```python
from build123d import *
from OCP.BRepFilletAPI import BRepFilletAPI_MakeChamfer

# Parameters (mm, degrees)
BOSS_EXTRUDE1_DEPTH       = 25.4
BOSS_EXTRUDE2_DEPTH       = 38.1
F_6_32_TAPPED_HOLE1_D     = 2.7051
F_6_32_TAPPED_HOLE1_DEPTH = 12.7
F_6_32_TAPPED_HOLE1_TIP   = 0.8126940302657266
CHAMFER1_SIZE             = 2.54
BOSS_EXTRUDE3_DEPTH       = 25.4
CHAMFER2_SIZE             = 7.619999999999999
CHAMFER2_SIZE2            = 5.388153672641502


with BuildPart() as part:
    # Sketch1 → Boss-Extrude1 (new body)
    with BuildSketch(Plane.XY):
        Polygon((0, -3.592102448427662), (-16.01038418160373, 12.418281733176066), (-16.010384181603733, 24.90038418160373), (16.01038418160373, 24.90038418160373), (16.010384181603733, 12.418281733176075), align=None)
        Polygon((0, 0), (-13.47038418160373, 13.47038418160373), (-13.470384181603732, 22.360384181603727), (13.470384181603732, 22.360384181603727), (13.47038418160373, 13.47038418160373), align=None, mode=Mode.SUBTRACT)
    extrude(amount=BOSS_EXTRUDE1_DEPTH)

    # Sketch2 → Boss-Extrude2 (add)
    with BuildSketch(Plane.XY.offset(25.4)):
        Polygon((0, 0), (-5.388153672641493, 5.388153672641493), (-7.184204896855324, 3.592102448427661), (0, -3.592102448427662), (7.184204896855322, 3.5921024484276627), (5.388153672641491, 5.3881536726414945), align=None)
    extrude(amount=BOSS_EXTRUDE2_DEPTH)

    # #6-32 Tapped Hole1
    with Locations(Plane(origin=(0, 24.90038418160373, 0), x_dir=(1, 0, 0), z_dir=(0, 1, 0))):
        with Locations((0, -3.175), (0, -22.225)):
            Hole(F_6_32_TAPPED_HOLE1_D / 2, depth=F_6_32_TAPPED_HOLE1_DEPTH)
            with Locations((0, 0, -(F_6_32_TAPPED_HOLE1_DEPTH + F_6_32_TAPPED_HOLE1_TIP / 2))):  # 118° drill point
                Cone(0, F_6_32_TAPPED_HOLE1_D / 2, F_6_32_TAPPED_HOLE1_TIP, mode=Mode.SUBTRACT)

    # Chamfer1
    chamfer1_edges = [part.edges().sort_by_distance(p)[0] for p in [
        (0, -3.592102448427662, 31.75),
    ]]
    chamfer(chamfer1_edges, length=CHAMFER1_SIZE)

    # Sketch5 → Boss-Extrude3 (add)
    with BuildSketch(Plane(origin=(0, 0, 0), x_dir=(-1, 0, 0), z_dir=(0, 0, -1))):
        Polygon((1.7960512242138398, -1.7960512242138225), (-1.7960512242138331, -1.7960512242138298), (-12.29, -1.796051224213831), (-12.289999999999996, -23.336051224213833), (-9.749999999999998, -23.336051224213833), (-9.749999999999998, -4.336051224213831), (9.749999999999998, -4.336051224213828), (9.750000000000005, -23.33605122421383), (12.290000000000003, -23.33605122421383), (12.29, -1.796051224213828), align=None)
    extrude(amount=-BOSS_EXTRUDE3_DEPTH)

    # Chamfer2: one chamfer whose edges measure the first distance from different faces: ONE call of the kernel's chamfer builder (chamfer() names one face for all edges)
    chamfer2_edges_1 = [part.edges().sort_by_distance(p)[0] for p in [
        (1.7960512242138322, -1.7960512242138291, 12.7),
    ]]
    chamfer2_side_1 = [part.faces().sort_by_distance(p)[0] for p in [
        (7.0430256121069155, -1.7960512242138404, 12.7),
    ]]
    chamfer2_edges_2 = [part.edges().sort_by_distance(p)[0] for p in [
        (-1.7960512242138293, -1.7960512242138293, 12.7),
    ]]
    chamfer2_side_2 = [part.faces().sort_by_distance(p)[0] for p in [
        (-7.043025612106914, -1.7960512242138118, 12.7),
    ]]
    chamfer2 = BRepFilletAPI_MakeChamfer(part.part.solid().wrapped)
    for e in chamfer2_edges_1:
        chamfer2.Add(CHAMFER2_SIZE, CHAMFER2_SIZE2, e.wrapped, chamfer2_side_1[0].wrapped)  # the first distance lies on this face
    for e in chamfer2_edges_2:
        chamfer2.Add(CHAMFER2_SIZE, CHAMFER2_SIZE2, e.wrapped, chamfer2_side_2[0].wrapped)  # the first distance lies on this face
    add(Compound.cast(chamfer2.Shape()), mode=Mode.REPLACE)


solid = part.part
```
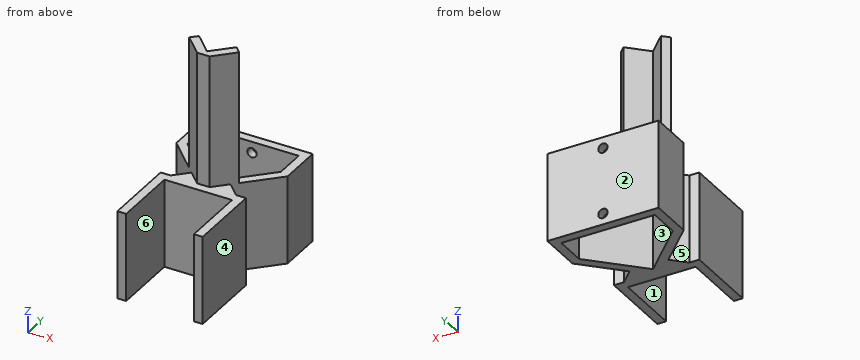
Input: part model. Units: mm. Frame: model coordinates. Face numbers are marked on the shaded views. A direction names the side the tool comes from. Coordinates: 2 decimals unless noted, no trailing zeros. Write each loop counter-clockwise with the first axis right and the second up, starting at its lowest first coordinate (ties: lowest second). Pieces come first, ordered by that corner, then holes. Notation, with made-up numbers: (-40, 89) -> (-35, 89) arc R27 ccw to (-35, 107) -> close; hole circle Ø3 at (-4.5, 34). An arc over 180 degrees is marked (long way). Answer as a JSON object with one key per item and string values.
1. Section B-B on z = 16. Return the cut outline in (x, y), then the cut area to 3 significant figures.
Result set:
{"outline": "(-16.01, 12.42) -> (-5.61, 2.01) -> (-9.42, -1.8) -> (-12.29, -1.8) -> (-12.29, -23.34) -> (-9.75, -23.34) -> (-9.75, -4.34) -> (9.75, -4.34) -> (9.75, -23.34) -> (12.29, -23.34) -> (12.29, -1.8) -> (9.42, -1.8) -> (5.61, 2.01) -> (16.01, 12.42) -> (16.01, 24.9) -> (-16.01, 24.9) -> close; hole (-13.47, 13.47) -> (0, 0) -> (13.47, 13.47) -> (13.47, 22.36) -> (-13.47, 22.36) -> close", "area": "420 mm2"}
2. Section D-D on z = 48. Return the cut outline in (x, y), then the cut area to 3 significant figures.
Result set:
{"outline": "(-7.18, 3.59) -> (-1.8, -1.8) -> (1.8, -1.8) -> (7.18, 3.59) -> (5.39, 5.39) -> (0, 0) -> (-5.39, 5.39) -> close", "area": "41.9 mm2"}
3. Material intervals for line 1 (Z direction, x = 0, y = 23.7); line 2 (Y direction, x = 9, z = 7); line 3 (X direction, y = -20, z = 8), sorted ascending. Write a range as from..to.
Result set:
{"line 1": "z = 0..1.82, 4.53..20.87, 23.58..25.4", "line 2": "y = -4.34..-1.38, 5.41..9, 22.36..24.9", "line 3": "x = -12.29..-9.75, 9.75..12.29"}
4. Access query for the marked faces 4, 5 and 6. Directions: +Z, -Z, +X, -X, +Y, -Y. A direction counts if a zero-diameter tool reaches every point of the face in a straight line with its end or side. Return the directions, or none.
Result set:
{"face 4": "+Z, -Z, +X, -Y", "face 5": "+Z, -Z, -X", "face 6": "+Z, -Z, -Y"}
5. Section A-A on y = -12.5. Return the cut outline in (x, z).
Result set:
{"outline": "(-12.29, 0) -> (-9.75, 0) -> (-9.75, 25.4) -> (-12.29, 25.4) -> close; (9.75, 0) -> (12.29, 0) -> (12.29, 25.4) -> (9.75, 25.4) -> close"}
6. Section C-C on x = -3.5. Return the cut outline in (y, z).
Result set:
{"outline": "(-4.34, 0) -> (3.5, 0) -> (3.5, 63.5) -> (-0.09, 63.5) -> (-0.09, 25.4) -> (-4.34, 25.4) -> close; (22.36, 0) -> (24.9, 0) -> (24.9, 25.4) -> (22.36, 25.4) -> close"}
7. Mould query, pull axis Y, two halves, no side actions, for the marked faces 1, 2 and 3. Classes: released by +Y, released by -Y, zero draft, split by the parting line, or undercut.
Result set:
{"face 1": "zero draft", "face 2": "released by +Y", "face 3": "undercut"}
8. First-contact query: P1, Ø12, axis at x = 7.5, z = 49, coming from the -Y side; P2, Ø12.5, axis at x = -1, z = 8, coming from the -Y side; P3, Ø6.5, axis at y = -12, z = 12.5, coming from the -X side. Flat tips, straight axial feed; report the tip coordinate or a pass-through.
Result set:
{"P1": "stops at y = -1.8", "P2": "stops at y = -4.34", "P3": "stops at x = -12.29"}
